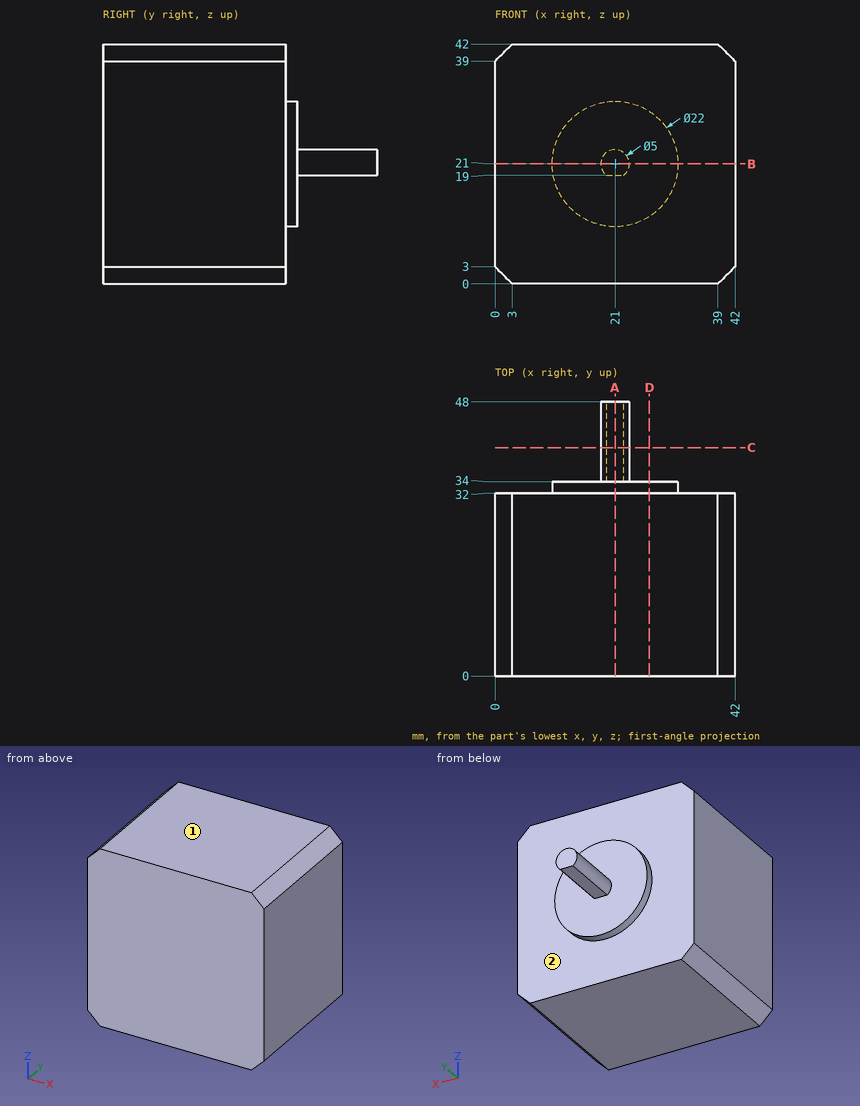
Check sheet for the drawn part. Datum: minimum x, y, z corner. Units: mm. A direction names the side the tool comes from. Coordinates: 2 decimals unless noted, no trailing zeros. Write each loop counter-clockwise with the first axis right and the second up, starting at its lowest first coordinate (ties: lowest second). Pieces come first, ordered by that corner, then holes. Notation, with made-up numbers: M 20,-37 L 41,-37 A28 cw 41,1 Z; hole C 76,0 d2. An arc over 180 degrees is marked long. One line per item, written item: value.
Item 1: Section check D-D, the plane x = 27. Record the boundary of the cut face in (y, z).
Check sheet entries:
outline: M 0,0 L 32,0 L 32,11.78 L 34,11.78 L 34,30.22 L 32,30.22 L 32,42 L 0,42 Z
Item 2: Section check B-B, the plane z = 21. Record the boundary of the cut face in (x, y).
Check sheet entries:
outline: M 0,0 L 42,0 L 42,32 L 32,32 L 32,34 L 23.5,34 L 23.5,48 L 18.5,48 L 18.5,34 L 10,34 L 10,32 L 0,32 Z
Item 3: Gauge pin test, flat ends, axial feed: pin 1 Ø8 at (x, z) = (14, 23.5) entering from -Y; pin 2 Ø3.5 at (x, y) = (21.5, 38.5) entering from -Z. Record the tip position at first contact, or that the pin passes through.
Check sheet entries:
pin 1: stops at y = 0
pin 2: stops at z = 19
Item 4: Section check C-C, the plane y = 40. Record the boundary of the cut face in (x, z).
Check sheet entries:
outline: M 19.5,19 L 22.5,19 A2.5 ccw long Z
Item 5: Scan lines: line 1 along Y through (x, z) = (11, 30.5); line 2 along Y through (x, z) = (17.5, 28.5); line 3 along Z through (x, y) = (20.5, 39). Record each from-to range of solid material in increasing order.
Check sheet entries:
line 1: y = 0 to 32
line 2: y = 0 to 34
line 3: z = 19 to 23.45
Item 6: Section check A-A, the plane x = 21. Record the boundary of the cut face in (y, z), plus the area to 3 significant figures.
Check sheet entries:
outline: M 0,0 L 32,0 L 32,10 L 34,10 L 34,19 L 48,19 L 48,23.5 L 34,23.5 L 34,32 L 32,32 L 32,42 L 0,42 Z
area: 1,450 mm^2
Item 7: Access from +Z, -Z, +X, -X, +Y, -Y to the whole of each face (thin tool, end or side, straight path). Record for the marked faces 1 and 2.
Check sheet entries:
face 1: +Z, +X, -X, +Y, -Y
face 2: +Y
